```python
from build123d import *

# Parameters (mm, degrees)
F0_W      = 35.2
F0_H      = 35.2
F1_DEPTH  = 7.7
F2_SIZE   = 6.1
F3_W      = 35.2
F3_H      = 35.2
F4_DEPTH  = 10
F5_SIZE   = 2.6
F7_DEPTH  = 11
F8_R      = 11
F9_DEPTH  = 2.3
F10_R     = 2.5
F11_DEPTH = 19
F12_W     = 5.253729
F12_H     = 0.933404
F13_DEPTH = 19
F14_R     = 1.5
F15_DEPTH = 6


with BuildPart() as f1:
    # F0 (on Top) → F1 (new body, symmetric)
    with BuildSketch(Plane.XY):
        Rectangle(F0_W, F0_H)
    extrude(amount=F1_DEPTH, both=True)

    # F2
    f2_edges = [f1.edges().sort_by_distance(p)[0] for p in [
        (-17.6, -17.6, 0),
        (17.6, -17.6, 0),
        (17.6, 17.6, 0),
        (-17.6, 17.6, 0),
    ]]
    chamfer(f2_edges, length=F2_SIZE)

    # F3 (on face) → F4 (join)
    with BuildSketch(Plane.XY.offset(7.7)):
        Rectangle(F3_W, F3_H)
    extrude(amount=F4_DEPTH)

    # F5
    f5_edges = [f1.edges().sort_by_distance(p)[0] for p in [
        (-17.6, -17.6, 12.7),
        (17.6, -17.6, 12.7),
        (17.6, 17.6, 12.7),
        (-17.6, 17.6, 12.7),
    ]]
    chamfer(f5_edges, length=F5_SIZE)

    # F6 (on face) → F7 (join)
    with BuildSketch(Plane(origin=(0, 0, -7.7), x_dir=(1, 0, 0), z_dir=(0, 0, -1))):
        Polygon((-15, -17.6), (15, -17.6), (17.6, -15), (17.6, 15), (15, 17.6), (-15, 17.6), (-17.6, 15), (-17.6, -15), align=None)
    extrude(amount=F7_DEPTH)

    # F8 (on face) → F9 (join)
    with BuildSketch(Plane.XY.offset(17.7)):
        Circle(F8_R)
    extrude(amount=F9_DEPTH)

    # F10 (on face) → F11 (join)
    with BuildSketch(Plane.XY.offset(20)):
        Circle(F10_R)
    extrude(amount=F11_DEPTH)

    # F12 (on face) → F13 (cut)
    with BuildSketch(Plane.XY.offset(39)):
        with Locations((-0.006502, 2.466702)):
            Rectangle(F12_W, F12_H)
    extrude(amount=-F13_DEPTH, mode=Mode.SUBTRACT)

    # F14 (on face) → F15 (cut)
    with BuildSketch(Plane.XY.offset(17.7)):
        with Locations((-13, 13)):
            Circle(F14_R)
        with Locations((13, 13)):
            Circle(F14_R)
        with Locations((-13, -13)):
            Circle(F14_R)
        with Locations((13, -13)):
            Circle(F14_R)
    extrude(amount=-F15_DEPTH, mode=Mode.SUBTRACT)


solid = f1.part
```
The listing builds one solid part. Answer for the finished solid, in the listing's coordinates (mm). A direction names the side the tool comes from. Coordinates: 2 decimals unless noted, no trailing zeros. Loops run counter-clockwise (first coordinate to the right, second up) from the corner with the lowest first, then second, coordinate; pieces in that order, holes last. Notation, with made-up numbers: (46.5, -28) - (94.5, -28) arc R27 cw to (94.5, -12) - close; hole circle Ø4 at (20, -14.5). An arc over 180 degrees is marked (long way). Use a Markdown table: item, result. Add a question column.
1) Given pin 1 (4 mm diameter, centred on x = 13, y = -13, fed in from +Z); pin 2 (1.5 mm diameter, centred on x = 13.5, y = -13, fed in from +Z); pin 3 (3.5 mm diameter, centred on x = 0, z = 34, fed in from +Y), each flat-ended and moving along its own axis, determine where each tip first touches the part or whether it passes through.
2) For faces 1 (the cylindrical face through (11.5, -12.93, 14.74)), 2 (the flat face through (15, 15, -7.7)), 3 (the flat face through (0, -17.6, 0)), 4 (the flat face through (-15, 15, -7.7)), 5 (the flat face through (16.3, -16.3, 12.6)), determine the directions among +Z, -Z, +X, -X, +Y, -Y from which every point of the face is accessible in a straight line to the end or side of a thin tool.
3) The part is cut by section D-D, the plane z = 23. Give the vertices of the cut face in (x, y), and give its area (3 significant figures).
4) Find the intervals of material crossed by line 1 (Y direction, x = -13, z = 15.55); line 2 (Z direction, x = 6.5, y = -3.5); line 3 (Z direction, x = 12, y = -10), in increasing order.
5) The part is cut by section A-A, the plane y = 13. Give the vertices of the cut face in (x, z).
6) The mould has two halves that part along X. Classify faces 6 (the flat face through (-15, -15, 7.7)), 7 (the flat face through (-14.5, -14.6, -0.1)), 8 (the flat face through (-13, -13, 11.7)), 9 (the flat face through (14.5, 14.6, 0.1)): released by +X, released by -X, zero draft, split by the parting line, or undercut.
7) The part is cut by section B-B, the plane x = 0. Give the vertices of the cut face in (y, z), and give its area (3 significant figures).
Here are the results:
| question | item | result |
|---|---|---|
| 1 | pin 1 | stops at z = 17.7 |
| 1 | pin 2 | stops at z = 11.7 |
| 1 | pin 3 | stops at y = 2 |
| 2 | face 1 | +Z |
| 2 | face 2 | +X, +Y |
| 2 | face 3 | +Z, -Z, +X, -X, -Y |
| 2 | face 4 | -X, +Y |
| 2 | face 5 | +Z, -Z, +X, -Y |
| 3 | outline | (-1.5, 2) arc R2.5 ccw (long way) to (1.5, 2) - close |
| 3 | area | 18.6 mm^2 |
| 4 | line 1 | y = -17.6 to -14.5, -11.5 to 11.5, 14.5 to 17.6 |
| 4 | line 2 | z = -18.7 to 20 |
| 4 | line 3 | z = -18.7 to 17.7 |
| 5 | outline | (-17.6, -18.7) - (17.6, -18.7) - (17.6, -7.7) - (16.1, -7.7) - (16.1, 7.7) - (17.6, 7.7) - (17.6, 17.7) - (14.5, 17.7) - (14.5, 11.7) - (11.5, 11.7) - (11.5, 17.7) - (-11.5, 17.7) - (-11.5, 11.7) - (-14.5, 11.7) - (-14.5, 17.7) - (-17.6, 17.7) - (-17.6, 7.7) - (-16.1, 7.7) - (-16.1, -7.7) - (-17.6, -7.7) - close |
| 6 | face 6 | zero draft |
| 6 | face 7 | released by -X |
| 6 | face 8 | undercut |
| 6 | face 9 | released by +X |
| 7 | outline | (-17.6, -18.7) - (17.6, -18.7) - (17.6, 17.7) - (11, 17.7) - (11, 20) - (2, 20) - (2, 39) - (-2.5, 39) - (-2.5, 20) - (-11, 20) - (-11, 17.7) - (-17.6, 17.7) - close |
| 7 | area | 1,420 mm^2 |
